```python
from build123d import *

# Parameters (mm, degrees)
SKETCH2_W                   = 60
SKETCH2_H                   = 20
BOSS_EXTRUDE1_DEPTH         = 6.35
M5_CLEARANCE_HOLE1_D        = 5.5
TAP_DRILL_FOR_M3X0_5_TAP1_D = 2.5
FILLET1_R                   = 7.5


with BuildPart() as part:
    # Sketch2 → Boss-Extrude1 (new body)
    with BuildSketch(Plane(origin=(0, 0, 0), x_dir=(1, 0, 0), z_dir=(0, 1, 0))):
        with Locations((30, 10)):
            Rectangle(SKETCH2_W, SKETCH2_H)
    extrude(amount=BOSS_EXTRUDE1_DEPTH)

    # M5 Clearance Hole1 (through all)
    with Locations(Plane(origin=(10, 6.35, -10), x_dir=(0, 0, 1), z_dir=(0, 1, 0))):
        with Locations((0, 0), (0, 15), (0, 30)):
            Hole(M5_CLEARANCE_HOLE1_D / 2)

    # Tap Drill for M3x0.5 Tap1 (through all)
    with Locations(Plane(origin=(55, 6.35, -10), x_dir=(0, 0, 1), z_dir=(0, 1, 0))):
        with Locations((0, 0)):
            Hole(TAP_DRILL_FOR_M3X0_5_TAP1_D / 2)

    # Fillet1
    fillet1_edges = [part.edges().sort_by_distance(p)[0] for p in [
        (0, 3.175, -20),
        (60, 3.175, -20),
        (60, 3.175, 0),
        (0, 3.175, 0),
    ]]
    fillet(fillet1_edges, radius=FILLET1_R)


solid = part.part
```
The listing builds one solid part. Answer for the finished solid, in the listing's coordinates (mm). Round coordinates to 2 decimals unless told otherwise and drop trailing zeros. Loops run counter-clockwise (first coordinate to the right, second up) from the corner with the lowest first, then second, coordinate; pieces in that order, holes last. Notation, with made-up numbers: (73.5, 89) - (125.5, 89) arc R15 ccw to (125.5, 114) - close; hole circle Ø7 at (-32, 14.25). An arc over 180 degrees is marked (long way). Return JSON: item names as keys, results as strings. Group by question number.
1. The mould has two halves that part along Z. Classify faces 1 (the cylindrical face through (27.727, 3.131, -9.642)), 2 (the cylindrical face through (2.139, 3.219, -2.255)), 3 (the flat face through (60, 3, -10)): pulls with the +Z half, pulls with the -Z half, needs draft (parallel to the pull), parting line crosses it, or undercut.
2. The part is cut by section D-D on z = -2. Determine the outline of the cut face in (x, y), then the cut area to 3 significant figures.
3. Consider probe 1 along X at (y, z) = (4.5, -10); probe 2 along X at (y, z) = (6, -11); probe 3 along X at (y, z) = (3.5, -4.75). Determine where each line is inside the solid, lowest interval first.
4. This flat-tipped pin is pushed along its axis until it touches: P1, Ø2, axis at y = 3, z = -16.5, coming from the +X side. Where does it stop, or does it pass through?
5. The part is cut by section C-C on y = 4.5. Determine the outline of the cut face in (x, z).
6. The part is cut by section B-B on z = -10. Determine the outline of the cut face in (x, y), then the cut area to 3 significant figures.
7. The part is cut by section A-A on x = 10. Determine the outline of the cut face in (y, z), then the cut area to 3 significant figures.
Resolved:
{
 "1": {"face 1": "undercut", "face 2": "pulls with the +Z half", "face 3": "needs draft"},
 "2": {"outline": "(2.4, 0) - (57.6, 0) - (57.6, 6.35) - (2.4, 6.35) - close", "area": "351 mm²"},
 "3": {"probe 1": "x = 0 to 7.25, 12.75 to 22.25, 27.75 to 37.25, 42.75 to 53.75, 56.25 to 60", "probe 2": "x = 0 to 7.44, 12.56 to 22.44, 27.56 to 37.44, 42.56 to 54.25, 55.75 to 60", "probe 3": "x = 0.52 to 59.48"},
 "4": {"P1": "stops at x = 59.37"},
 "5": {"outline": "(0, -12.5) arc R7.5 ccw to (7.5, -20) - (52.5, -20) arc R7.5 ccw to (60, -12.5) - (60, -7.5) arc R7.5 ccw to (52.5, 0) - (7.5, 0) arc R7.5 ccw to (0, -7.5) - close; hole circle Ø5.5 at (10, -10); hole circle Ø5.5 at (25, -10); hole circle Ø5.5 at (40, -10); hole circle Ø2.5 at (55, -10)"},
 "6": {"outline": "(0, 0) - (7.25, 0) - (7.25, 6.35) - (0, 6.35) - close; (12.75, 0) - (22.25, 0) - (22.25, 6.35) - (12.75, 6.35) - close; (27.75, 0) - (37.25, 0) - (37.25, 6.35) - (27.75, 6.35) - close; (42.75, 0) - (53.75, 0) - (53.75, 6.35) - (42.75, 6.35) - close; (56.25, 0) - (60, 0) - (60, 6.35) - (56.25, 6.35) - close", "area": "260 mm²"},
 "7": {"outline": "(0, -20) - (6.35, -20) - (6.35, -12.75) - (0, -12.75) - close; (0, -7.25) - (6.35, -7.25) - (6.35, 0) - (0, 0) - close", "area": "92.1 mm²"}
}
